Autodesk Inventor part; units mm, degrees
ref_plane "YZ Plane" through (0, 0, 0) normal (1, 0, 0) x (0, 1, 0)
ref_plane "XZ Plane" through (0, 0, 0) normal (0, 1, 0) x (-1, 0, 0)
ref_plane "XY Plane" through (0, 0, 0) normal (0, 0, 1) x (1, 0, 0)
sketch "Sketch4" plane through (0, 0, 0) normal (0, 1, 0) x (-1, 0, 0)
  line L0 (-70, 73) -> (70, 73)
  line L1 (70, -73) -> (-70, -73)
  line L2 (-70, -73) -> (-70, 73)
  line L3 (-66, -69) -> (70, -69)
  line L4 (70, 69) -> (-66, 69)
  line L5 (-66, 69) -> (-66, -69)
  line L6 (70, 73) -> (70, 69)
  line L7 (70, -69) -> (70, -73)
  point P0 (0, 0)
  point P1 (-66, 65)
  dimension "Housing_Length" = 140
  dimension "Housing_Width" = 146
  dimension "d15" = 4
  dimension "d36" = 136
  dimension "d37" = 138
extrude "Extrusion4" add sketch "Sketch4" along normal blind 95
sketch "Sketch6" plane through (0, 95, 0) normal (0, 1, 0) x (1, 0, 0)
  line L0 (70, 73) -> (-70, 73)
  line L1 (-70, -69) -> (-70, -73)
  line L2 (70, 73) -> (-70, 73)
  line L3 (-70, 73) -> (-70, -73)
  line L4 (-70, -73) -> (70, -73)
  line L5 (70, -73) -> (70, 73)
  line L6 (62, -65) -> (-70, -65)
  line L7 (-70, 65) -> (62, 65)
  line L8 (62, 65) -> (62, -65)
  point P0 (0, 0)
  dimension "Lip_Width" = 8
extrude "Extrusion5" add sketch "Sketch6" against normal blind 5 contours L5 L4 L1 L3 L6 L8 L7 L0
sketch "Sketch10" plane through (0, 0, 0) normal (0, -1, 0) x (1, 0, 0)
  line L0 (66, -69) -> (66, 69)
  circle A0 centre (-70, 0) radius 135
  circle A1 centre (-70, 0) radius 110
  line L1 (-70, 73) -> (70, 73)
  line L2 (12.2861, 73) -> (70, 73)
  line L3 (70, -73) -> (-70, -73)
  line L4 (70, 73) -> (70, -73)
  line L5 (70, -73) -> (12.2861, -73)
  circle A2 centre (-70, 0) radius 127.5
  line L6 (-70, 0) -> (-70, 135)
  circle A3 centre (-70, 127.5) radius 2.75
  circle A4 centre (-144.9426, 103.1497) radius 2.75
  circle A5 centre (-191.2597, 39.3997) radius 2.75
  circle A6 centre (-191.2597, -39.3997) radius 2.75
  circle A7 centre (-144.9426, -103.1497) radius 2.75
  circle A8 centre (-70, -127.5) radius 2.75
  circle A9 centre (4.9426, -103.1497) radius 2.75
  circle A10 centre (51.2597, -39.3997) radius 2.75
  circle A11 centre (51.2597, 39.3997) radius 2.75
  circle A12 centre (4.9426, 103.1497) radius 2.75
  point P0 (0, 0)
  dimension "d52" = 270
  dimension "d57" = 255
  dimension "d53" = 136
  dimension "d54" = 220
  dimension "d58" = 5.5
  dimension "d61" = 360
extrude "Extrusion9" add sketch "Sketch10" against normal blind 1 contours A0 L3 A2 A10 A11 L1 | A0 L1 L4 L3 | A2 A11 A10 L3 A1 L1
properties part number "Galvo Housing-01"
CAD build for the part. Positions are in the model's coordinates, mm. A direction names the side the tool comes from. Round coordinates to 2 decimals unless told otherwise and drop trailing zeros. Loops run counter-clockwise (first coordinate to the right, second up) from the corner with the lowest first, then second, coordinate; pieces in that order, holes last.
(1) Which spindle directions (+Z, -Z, +X, -X, +Y, -Y) get a long thin tool onto all of the face, cutting with end or side? Do faces 1 (the flat face through (46, 1, 1)), 2 (the cylindrical face through (50.902, 0.493, -36.673)), 3 (the flat face through (-3, 93, 65)). Say none if no direction does.
(2) Cut at B-B (y = 83). Give the cut face in (x, z).
(3) Two-plate mould, pull along Z, no slides. Class faces 4 (the flat face through (63, 95, 6)), 5 (the flat face through (66, 45, 1)), 6 (the flat face through (1, 47, 73)): +Z half, -Z half, draft (parallel to the pull), parting line (faces both ways), or undercut.
(4) Cut at D-D (z = -30). Give the cut face in (x, y), plus the area to 3 significant figures.
(5) Cut at C-C (x = 59.5). Give the cut face in (y, z).
(6) Cut at A-A (x = -61). Give the cut face in (y, z).
(7) Wall check: line 1 along Z through (x, y) = (19.5, 51); line 2 along X through (y, z) = (42.5, 27.5); line 3 along Y through (x, z) = (56.5, 43). Give the ranges that are in metal, low to high.
(8) Drop flat-ended pins along their axis: pin 1 (1 mm diameter, centred on y = 61, z = 14, fed in from -X); pin 2 (1.5 mm diameter, centred on y = 93.5, z = -24.5, fed in from -X); pin 3 (4.5 mm diameter, centred on x = 51.26, z = -39.4, fed in from +Y). Give the stop position or say it passes through.
Findings below:
1. face 1: -X
1. face 2: +Y, -Y
1. face 3: -X, +Y
2. outline: (-70, -73) - (70, -73) - (70, 73) - (-70, 73) - (-70, 69) - (66, 69) - (66, -69) - (-70, -69) - close
3. face 4: draft
3. face 5: undercut
3. face 6: +Z half
4. outline: (35.83, 0) - (70, 0) - (70, 95) - (62, 95) - (62, 90) - (66, 90) - (66, 1) - (35.83, 1) - close
4. area: 430 mm2
5. outline: (0, -73) - (95, -73) - (95, -65) - (90, -65) - (90, -69) - (1, -69) - (1, 69) - (90, 69) - (90, 65) - (95, 65) - (95, 73) - (0, 73) - close
6. outline: (0, -73) - (95, -73) - (95, -65) - (90, -65) - (90, -69) - (0, -69) - close; (0, 69) - (90, 69) - (90, 65) - (95, 65) - (95, 73) - (0, 73) - close
7. line 1: z = -73 to -69, 69 to 73
7. line 2: x = 66 to 70
7. line 3: y = 0 to 1
8. pin 1: stops at x = 66
8. pin 2: stops at x = 62
8. pin 3: passes through
